```python
from build123d import *

# Parameters (mm, degrees)
SKETCH1_R           = 11
SKETCH1_R_2         = 1.75
BOSS_EXTRUDE1_DEPTH = 3
BOSS_EXTRUDE2_DEPTH = 3.1
BOSS_EXTRUDE3_DEPTH = 2.6
FILLET1_R           = 3
FILLET2_R           = 3


with BuildPart() as part:
    # Sketch1 → Boss-Extrude1 (new body)
    with BuildSketch(Plane.XY):
        Polygon((0, 46.4), (5, 51.4), (45.25, 51.4), (50.25, 46.4), (50.25, 0), (0, 0), align=None)
        with Locations((25.125, 30.4)):
            Circle(SKETCH1_R, mode=Mode.SUBTRACT)
        with Locations((9.625, 45.9)):
            Circle(SKETCH1_R_2, mode=Mode.SUBTRACT)
        with Locations((40.625, 45.9)):
            Circle(SKETCH1_R_2, mode=Mode.SUBTRACT)
        with Locations((40.625, 14.9)):
            Circle(SKETCH1_R_2, mode=Mode.SUBTRACT)
        with Locations((9.625, 14.9)):
            Circle(SKETCH1_R_2, mode=Mode.SUBTRACT)
    extrude(amount=BOSS_EXTRUDE1_DEPTH)

    # Sketch2 → Boss-Extrude2 (add)
    with BuildSketch(Plane.XZ):
        Polygon((0, 3), (50.25, 3), (50.25, -45.4), (45.25, -50.4), (5, -50.4), (0, -45.4), align=None)
        with BuildLine():
            Line((42.15, -9.1), (42.15, -39.1))
            ThreePointArc((42.15, -39.1), (40.15, -41.1), (38.15, -39.1))
            Line((38.15, -39.1), (38.15, -9.1))
            ThreePointArc((38.15, -9.1), (40.15, -7.1), (42.15, -9.1))
        make_face(mode=Mode.SUBTRACT)
        with BuildLine():
            Line((8.1, -9.1), (8.1, -39.1))
            ThreePointArc((8.1, -39.1), (10.1, -41.1), (12.1, -39.1))
            Line((12.1, -39.1), (12.1, -9.1))
            ThreePointArc((12.1, -9.1), (10.1, -7.1), (8.1, -9.1))
        make_face(mode=Mode.SUBTRACT)
    extrude(amount=-BOSS_EXTRUDE2_DEPTH)

    # Sketch3 → Boss-Extrude3 (add)
    with BuildSketch(Plane.ZY):
        Polygon((0, 25.8), (-17.2, 3.1), (-17.2, 0), (3, 0), (3, 25.8), align=None)
    boss_extrude3 = extrude(amount=-BOSS_EXTRUDE3_DEPTH)

    # Mirror1: Boss-Extrude3 across plane
    add(boss_extrude3.mirror(Plane.ZY.offset(-25.125)))

    # Fillet1
    fillet1_edges = [part.edges().sort_by_distance(p)[0] for p in [
        (25.125, 0, 3),
    ]]
    fillet(fillet1_edges, radius=FILLET1_R)

    # Fillet2
    fillet2_edges = [part.edges().sort_by_distance(p)[0] for p in [
        (25.125, 3.1, 0),
    ]]
    fillet(fillet2_edges, radius=FILLET2_R)


solid = part.part
```
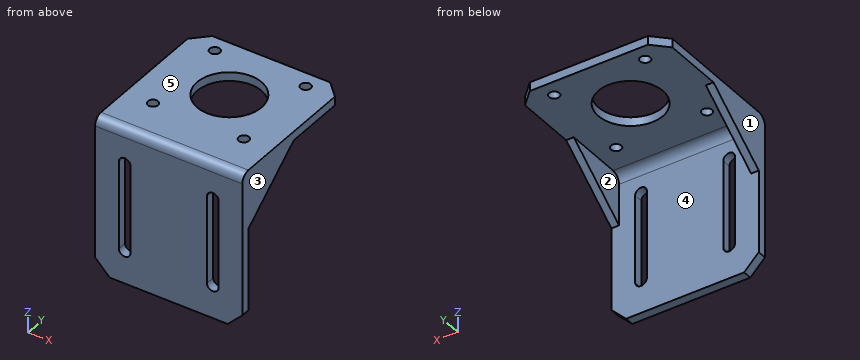
The model under review builds one solid part; all positions refer to its coordinate system, in mm. Face numbers are marked on the shaded views. A direction names the side the tool comes from. Round coordinates to 2 decimals unless told otherwise and drop trailing zeros. Write each loop counter-clockwise with the first axis right and the second up, starting at its lowest first coordinate (ties: lowest second). Pieces come first, ordered by that corner, then holes.
(1) Insertion check: pin 1 (19 mm diameter, centred on y = 19.5, z = -6.5, fed in from -X); pin 2 (23.5 mm diameter, centred on x = 25, z = -37, fed in from +Y); pin 3 (2 mm diameter, centred on x = 7, y = 42.5, fed in from -Z); pin 4 (3 mm diameter, centred on x = 9.625, y = 45.9, fed in from +Z). Each pin has a flat end and moves straight along its axis. Give the tip position at first contact, or say it passes through.
(2) We need section A-A on y = 30.4. Give the boundary of the cut face in (x, z) (3 decimals).
(3) Mouldability with a two-part tool opening along X and no side actions: class the marked faces 1, 2 and 3 as +X half, -X half, draft (parallel to the pull), parting line (faces both ways), or undercut.
(4) Wall thickness on L1, parallel to Y at x = 28.5, z = -41; L2, parallel to Z at x = 14, y = 27; L3, parallel to Z at x = 48.5, y = 11.5: over which ranges is each line inside the solid? List them lowest first.
(5) We need section C-C on x = 17. Give the boundary of the cut face in (y, z), and give its area (3 significant figures).
(6) We need section D-D on y = 14.9. Give the boundary of the cut face in (x, z) (3 decimals), and give its area (3 significant figures).
(7) Machinability: for the marked faces 4 and 5, which of the approach directions +Z, -Z, +X, -X, +Y, -Y give a long, thin tool a straight path to every point of the face, cutting with its end or side? Answer none if there is none.
(8) We need section B-B on z = -32. Give the boundary of the cut face in (x, y), and give its area (3 significant figures).
Findings below:
1. pin 1: stops at x = 0
1. pin 2: stops at y = 3.1
1. pin 3: stops at z = 0
1. pin 4: passes through
2. outline: (0, 0) - (14.125, 0) - (14.125, 3) - (0, 3) - close; (36.125, 0) - (50.25, 0) - (50.25, 3) - (36.125, 3) - close
3. face 1: -X half
3. face 2: undercut
3. face 3: +X half
4. L1: y = 0 to 3.1
4. L2: z = 0 to 3
4. L3: z = -10.84 to 3
5. outline: (0, -50.4) - (3.1, -50.4) - (3.1, -3) arc R3 cw to (6.1, 0) - (22.98, 0) - (22.98, 3) - (3, 3) arc R3 ccw to (0, 0) - close; (37.82, 0) - (51.4, 0) - (51.4, 3) - (37.82, 3) - close
5. area: 266 mm2
6. outline: (0, -8.259) - (2.6, -8.259) - (2.6, 0) - (7.875, 0) - (7.875, 3) - (0, 3) - close; (11.375, 0) - (38.875, 0) - (38.875, 3) - (11.375, 3) - close; (42.375, 0) - (47.65, 0) - (47.65, -8.259) - (50.25, -8.259) - (50.25, 3) - (42.375, 3) - close
6. area: 173 mm2
7. face 4: -Z, +Y
7. face 5: +Z, +X, -X, +Y, -Y
8. outline: (0, 0) - (8.1, 0) - (8.1, 3.1) - (0, 3.1) - close; (12.1, 0) - (38.15, 0) - (38.15, 3.1) - (12.1, 3.1) - close; (42.15, 0) - (50.25, 0) - (50.25, 3.1) - (42.15, 3.1) - close
8. area: 131 mm2
